Geometry: final body of the model. Coordinates: model frame, mm. Give positions to 0.01 mm unless a question says otherwise; leave off trailing zeros. Order: outer loops, then holes, each group sorted by start corner. A loop starts at its lowest first (then second) coordinate and runs counter-clockwise, first axis right, second up. Notation, with made-up numbers: (42, 20.25) -> (100, 20.25) arc R29 cw to (100, 57.25) -> close; hole circle Ø9 at (71, 1). An arc over 180 degrees is marked (long way). One line per item, written item: value. Start each with the question number.
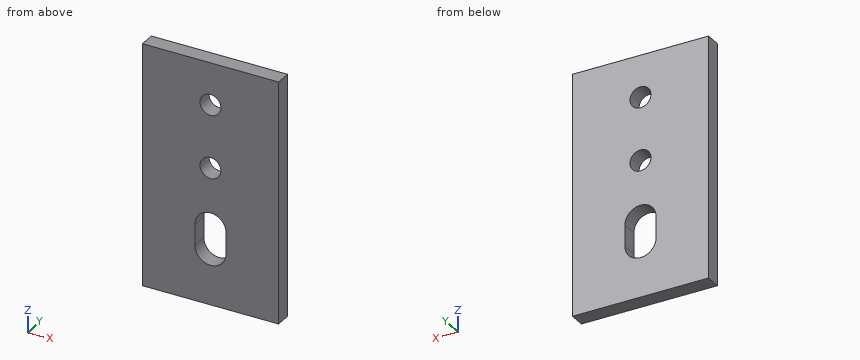
```python
from build123d import *

# Parameters (mm, degrees)
SKETCH1_W           = 13
SKETCH1_H           = 23
SKETCH1_R           = 1
BOSS_EXTRUDE1_DEPTH = 1.5


with BuildPart() as part:
    # Sketch1 → Boss-Extrude1 (new body)
    with BuildSketch(Plane(origin=(0, 0, 0), x_dir=(1, 0, 0), z_dir=(0, 1, 0))):
        Rectangle(SKETCH1_W, SKETCH1_H)
        with Locations(Location((0, -1.5, 0), (0, 0, 270))):
            Circle(SKETCH1_R, mode=Mode.SUBTRACT)
        with Locations(Location((0, -7.5, 0), (0, 0, 270))):
            Circle(SKETCH1_R, mode=Mode.SUBTRACT)
        with BuildLine():
            Line((-1.493243243, 4.25), (-1.493243243, 6.25))
            ThreePointArc((-1.493243243, 6.25), (0, 7.743243243), (1.493243243, 6.25))
            Line((1.493243243, 6.25), (1.493243243, 4.25))
            ThreePointArc((1.493243243, 4.25), (0, 2.756756757), (-1.493243243, 4.25))
        make_face(mode=Mode.SUBTRACT)
    extrude(amount=BOSS_EXTRUDE1_DEPTH)


solid = part.part
```
1. Cut plane B-B, the plane x = 0. Return loops of the section in (y, z).
2. Cut plane C-C, the plane y = 1.1. Return loops of the section in (x, z), then the cut area to 3 significant figures.
3. Cut plane D-D, the plane z = -5.5. Return loops of the section in (x, y).
4. Pin query (flat end, axial travel): P1, Ø1.8, axis at x = 0, z = 1.5, coming from the -Y side. Return the tip coordinate at first contact, or that it passes through.
5. Material intervals for L1, parallel to X at y = 1.25, z = 1.5; L2, parallel to Z at x = -0.5, y = 1; L3, parallel to X at y = 0.55, z = -6, sorted ascending. Write a range as [from, to].
6. Cut plane A-A, the plane z = 1.5. Return loops of the section in (x, y).
Answers follow:
1. outline: (0, -11.5) -> (1.5, -11.5) -> (1.5, -7.74) -> (0, -7.74) -> close; (0, -2.76) -> (1.5, -2.76) -> (1.5, 0.5) -> (0, 0.5) -> close; (0, 2.5) -> (1.5, 2.5) -> (1.5, 6.5) -> (0, 6.5) -> close; (0, 8.5) -> (1.5, 8.5) -> (1.5, 11.5) -> (0, 11.5) -> close
2. outline: (-6.5, -11.5) -> (6.5, -11.5) -> (6.5, 11.5) -> (-6.5, 11.5) -> close; hole (-1.49, -6.25) arc R1.49 ccw to (1.49, -6.25) -> (1.49, -4.25) arc R1.49 ccw to (-1.49, -4.25) -> close; hole circle Ø2 at (0, 1.5); hole circle Ø2 at (0, 7.5)
2. area: 280 mm²
3. outline: (-6.5, 0) -> (-1.49, 0) -> (-1.49, 1.5) -> (-6.5, 1.5) -> close; (1.49, 0) -> (6.5, 0) -> (6.5, 1.5) -> (1.49, 1.5) -> close
4. P1: passes through
5. L1: x = [-6.5, -1], [1, 6.5]
5. L2: z = [-11.5, -7.66], [-2.84, 0.63], [2.37, 6.63], [8.37, 11.5]
5. L3: x = [-6.5, -1.49], [1.49, 6.5]
6. outline: (-6.5, 0) -> (-1, 0) -> (-1, 1.5) -> (-6.5, 1.5) -> close; (1, 0) -> (6.5, 0) -> (6.5, 1.5) -> (1, 1.5) -> close
